Model file for the job. Use its own axes, mm. A direction names the side the tool comes from. Coordinates: 2 decimals unless noted, no trailing zeros. Write each loop counter-clockwise with the first axis right and the second up, starting at its lowest first coordinate (ties: lowest second). Pieces come first, ordered by that corner, then holes.
Q1. Pin check, flat tips, straight feed: P1, Ø4.5, axis at x = -3.5, y = 14, coming from the -Z side; P2, Ø8, axis at x = 7.5, y = 22, coming from the +Z side; P3, Ø1.9, axis at x = 1.5, z = -6, coming from the -Y side. Stop position of each tip, or through.
Q2. Pull direction X, two halves, no side cores. Call faces 4 (the cylindrical face through (-10.59, 14.08, 28.79)), 5 (the flat face through (4, 2, 19)), 6 (the flat face through (0, 29, 7)), 7 (the flat face through (-5, 8, -4)): released by +X, released by -X, zero draft, split by the parting line, or undercut.
Q3. Drill centre lines: probe 1 along X at (y, z) = (1.55, 17); probe 2 along X at (y, z) = (8.75, 17); probe 3 along Z at (x, y) = (2.5, 12.5). Where is each one in solid material? Low to high.
Q4. Which spindle directions (+Z, -Z, +X, -X, +Y, -Y) get a long thin tool onto all of the face, cutting with end or side? Do faces 1 (the cylindrical face through (10.61, 14.08, 28.77)), 2 (the cylindrical face through (0.345, 28.24, 24.842)), 3 (the cylindrical face through (-0.369, 15.673, 3.275)). Say none if no direction does.
Q5. Band-saw the part on A-A, the plane z = -2. Write the cut outline in (x, y).
Q6. Band-saw the part on C-C, the plane y = 8.15. State how many separate pieces and enclosed holes the cut face has, plus the area to 3 significant figures.
Q7. Band-saw the part on B-B, the plane z = 17. Write the cut outline in (x, y), plus the area to 3 significant figures.
Autodesk Inventor part; units mm, degrees
ref_plane "2DUMMY_XY" through (0, 14.5, 0) normal (0, 0, -1) x (1, 0, 0)
ref_plane "2DUMMY_YZ" through (0, 14.5, 0) normal (1, 0, 0) x (0, -1, 0)
ref_plane "2DUMMY_ZX" through (0, 14.5, 0) normal (0, -1, 0) x (0, 0, -1)
sketch "Sketch_2" plane through (0, 0, 0) normal (1, 0, 0) x (0, 1, 0)
  line L0 (0, 29.5) -> (0, 0)
  line L1 (0, 0) -> (29, 0)
  line L2 (29, 0) -> (29, 27.5198)
  arc A0 (29, 27.5198) -> (27.5262, 29.0195) centre (27.5, 27.5198) ccw
  line L3 (27.5262, 29.0195) -> (0, 29.5)
extrude "Extrusion1" add sketch "Sketch_2" along normal mid plane 22
sketch "Sketch_3" plane through (0, 0, 0) normal (0, 0.9998, -0.0175) x (1, 0, 0)
  line L0 (-11, -28) -> (-11, -38)
  line L1 (-11, -38) -> (11, -38)
  line L2 (11, -38) -> (11, -28)
  arc A0 (9.5, -29.5) -> (11, -28) centre (9.5, -28) ccw
  line L3 (9.5, -29.5) -> (-9.5, -29.5)
  arc A1 (-11, -28) -> (-9.5, -29.5) centre (-9.5, -28) ccw
extrude "Extrusion2" cut sketch "Sketch_3" along normal mid plane 60
sketch "Sketch_4" plane through (0, 0, 0) normal (0, 0, 1) x (1, 0, 0)
  arc A0 (-9.5, 29) -> (-11, 27.5) centre (-9.5, 27.5) ccw
  line L0 (-9.5, 29) -> (9.5, 29)
  arc A1 (11, 27.5) -> (9.5, 29) centre (9.5, 27.5) ccw
  line L1 (11, 27.5) -> (11, 37.5)
  line L2 (11, 37.5) -> (-11, 37.5)
  line L3 (-11, 37.5) -> (-11, 27.5)
extrude "Extrusion3" cut sketch "Sketch_4" along normal blind 29.5
sketch "Sketch_5" plane through (0, 0, 0) normal (1, 0, 0) x (0, 1, 0)
  line L0 (0, 17) -> (29, 17)
  line L1 (29, 17) -> (29, 9.15)
  line L2 (29, 9.15) -> (27.5, 9.15)
  line L3 (27.5, 9.15) -> (27.5, 13)
  line L4 (27.5, 13) -> (2, 13)
  line L5 (2, 13) -> (2, 9.15)
  line L6 (2, 9.15) -> (0, 9.15)
  line L7 (0, 9.15) -> (0, 17)
  line L8 (0, 17) -> (29, 17)
revolve "Revolution1" cut sketch "Sketch_5" angle 360 about axis through (0, 0, 17) along (0, -1, 0)
sketch "Sketch_16" plane through (0, 0, 0) normal (0, 0, 1) x (1, 0, 0)
  arc A0 (-7.85, 3.5) -> (-6.35, 2) centre (-6.35, 3.5) ccw
  line L0 (-6.35, 2) -> (6.35, 2)
  arc A1 (6.35, 2) -> (7.85, 3.5) centre (6.35, 3.5) ccw
  line L1 (7.85, 3.5) -> (7.85, 24.1)
  arc A2 (7.85, 24.1) -> (6.35, 25.6) centre (6.35, 24.1) ccw
  line L2 (6.35, 25.6) -> (-6.35, 25.6)
  arc A3 (-6.35, 25.6) -> (-7.85, 24.1) centre (-6.35, 24.1) ccw
  line L3 (-7.85, 24.1) -> (-7.85, 3.5)
extrude "Extrusion4" cut sketch "Sketch_16" along normal blind 0.1
sketch "Sketch6" plane through (0, 0, 0.1) normal (0, 0, -1) x (-1, 0, 0)
  point P0 (0, 14.5)
hole "Hole1" at (0, 14.5, 0.1) direction (0, 0, 1) diameter 2.459 depth 6 tip angle 120 countersink diameter 3 countersink angle 90
sketch "Sketch_18" plane through (0, 0, 0) normal (1, 0, 0) x (0, 1, 0)
  line L0 (23.4, 0.1) -> (22.6, 0.1)
  line L1 (22.6, 0.1) -> (22.6, -10.5)
  line L2 (22.6, -10.5) -> (22.8, -11.5)
  line L3 (22.8, -11.5) -> (23.2, -11.5)
  line L4 (23.2, -11.5) -> (23.4, -10.5)
  line L5 (23.4, -10.5) -> (23.4, 0.1)
extrude "Extrusion5" add sketch "Sketch_18" along normal mid plane 6.3
sketch "Sketch_7" plane through (0, 8.5, 0) normal (0, 1, 0) x (1, 0, 0)
  line L0 (5, 8.5) -> (5, -0.1)
  line L1 (5, -0.1) -> (5.8, -0.1)
  line L2 (5.8, -0.1) -> (5.8, 8.5)
  line L3 (5.8, 8.5) -> (5.6, 9.5)
  line L4 (5.6, 9.5) -> (5.2, 9.5)
  line L5 (5.2, 9.5) -> (5, 8.5)
extrude "Extrusion6" add sketch "Sketch_7" along normal mid plane 6.3
sketch "Sketch_8" plane through (0, 8.5, 0) normal (0, 1, 0) x (1, 0, 0)
  line L0 (-5.8, 8.5) -> (-5.8, -0.1)
  line L1 (-5.8, -0.1) -> (-5, -0.1)
  line L2 (-5, -0.1) -> (-5, 8.5)
  line L3 (-5, 8.5) -> (-5.2, 9.5)
  line L4 (-5.2, 9.5) -> (-5.6, 9.5)
  line L5 (-5.6, 9.5) -> (-5.8, 8.5)
extrude "Extrusion7" add sketch "Sketch_8" along normal mid plane 6.3
sketch "Sketch_10" plane through (0, 0, 0) normal (0, 1, 0) x (-1, 0, 0)
  circle A0 centre (0, -7.5) radius 0.65
extrude "Extrusion8" cut sketch "Sketch_10" along normal blind 29
sketch "Sketch_11" plane through (0, 0, 0) normal (1, 0, 0) x (0, 1, 0)
  circle A0 centre (8.15, -6.1) radius 0.65
extrude "Extrusion9" cut sketch "Sketch_11" along normal mid plane 22
sketch "Sketch_12" plane through (0, 0, 0) normal (0, 1, 0) x (-1, 0, 0)
  line L0 (3.15, -10.5) -> (1.7358, -11.9142)
  line L1 (1.7358, -11.9142) -> (-1.7358, -11.9142)
  line L2 (-1.7358, -11.9142) -> (-3.15, -10.5)
  line L3 (-3.15, -10.5) -> (-3.15, -12.5)
  line L4 (-3.15, -12.5) -> (3.15, -12.5)
  line L5 (3.15, -12.5) -> (3.15, -10.5)
extrude "Extrusion10" cut sketch "Sketch_12" along normal blind 29
sketch "Sketch_13" plane through (0, 0, 0) normal (1, 0, 0) x (0, 1, 0)
  line L0 (11.65, -8.5) -> (10.2358, -9.9142)
  line L1 (10.2358, -9.9142) -> (6.7642, -9.9142)
  line L2 (6.7642, -9.9142) -> (5.35, -8.5)
  line L3 (5.35, -8.5) -> (5.35, -10.5)
  line L4 (5.35, -10.5) -> (11.65, -10.5)
  line L5 (11.65, -10.5) -> (11.65, -8.5)
extrude "Extrusion11" cut sketch "Sketch_13" along normal mid plane 22
ref_plane "2DUMMY_XY" through (0, 14.5, 0) normal (0, 0, -1) x (1, 0, 0)
ref_plane "2DUMMY_YZ" through (0, 14.5, 0) normal (1, 0, 0) x (0, -1, 0)
ref_plane "2DUMMY_ZX" through (0, 14.5, 0) normal (0, -1, 0) x (0, 0, -1)
ref_plane "ANBAU_Stecker_XY" through (0, 14.5, 0) normal (0, 0, 1) x (1, 0, 0)
ref_plane "ANBAU_Stecker_YZ" through (0, 14.5, 0) normal (1, 0, 0) x (0, 1, 0)
ref_plane "ANBAU_Stecker_ZX" through (0, 14.5, 0) normal (0, 1, 0) x (0, 0, 1)
ref_plane "IP1_XY" through (0, 27.5, 17) normal (0, -1, 0) x (1, 0, 0)
ref_plane "IP1_YZ" through (0, 27.5, 17) normal (1, 0, 0) x (0, 0, 1)
ref_plane "IP1_ZX" through (0, 27.5, 17) normal (0, 0, 1) x (0, -1, 0)
properties part number "389924 MSFG-24-42-50/60---(P)"
Answer sheet:
1. P1: stops at z = 0.1
1. P2: stops at z = 29.19
1. P3: stops at y = 22.6
2. face 4: released by -X
2. face 5: undercut
2. face 6: zero draft
2. face 7: undercut
3. probe 1: x = -11 to -7.85, 7.85 to 11
3. probe 2: x = -11 to -4, 4 to 11
3. probe 3: z = 0.1 to 13.88, 20.12 to 29.28
4. face 1: +Z, +X, +Y
4. face 2: +Y
4. face 3: -Z
5. outline: (-5.8, 5.35) - (-5, 5.35) - (-5, 11.65) - (-5.8, 11.65) - close; (-3.15, 22.6) - (3.15, 22.6) - (3.15, 23.4) - (-3.15, 23.4) - close; (5, 5.35) - (5.8, 5.35) - (5.8, 11.65) - (5, 11.65) - close
6. separate pieces: 3
6. enclosed holes: 1
6. area: 606 mm2
7. outline: (-11, 0) - (-7.85, 0) - (-7.85, 2) - (-4, 2) - (-4, 27.5) - (-7.85, 27.5) - (-7.85, 29) - (-9.5, 29) arc R1.5 ccw to (-11, 27.5) - close; (4, 2) - (7.85, 2) - (7.85, 0) - (11, 0) - (11, 27.5) arc R1.5 ccw to (9.5, 29) - (7.85, 29) - (7.85, 27.5) - (4, 27.5) - close
7. area: 378 mm2
